from build123d import *

# Parameters (mm, degrees)
F0_R     = 25.4
F1_DEPTH = 12.7
F2_W     = 4.56177
F2_H     = 5.815812
F3_DEPTH = 12.701
F4_R     = 4.759949
F5_DEPTH = 12.701


with BuildPart() as f1:
    # F0 (on Top) → F1 (new body)
    with BuildSketch(Plane.XY):
        Circle(F0_R)
    extrude(amount=F1_DEPTH)

    # F2 (on face) → F3 (cut, through all)
    with BuildSketch(Plane.XY.offset(12.7)):
        with Locations((-10.897615, -5.573769)):
            Rectangle(F2_W, F2_H)
    extrude(amount=-F3_DEPTH, mode=Mode.SUBTRACT)

    # F4 (on face) → F5 (cut, through all)
    with BuildSketch(Plane(origin=(0, 0, 0), x_dir=(1, 0, 0), z_dir=(0, 0, -1))):
        with Locations((8.635784, 2.300633)):
            Circle(F4_R)
    extrude(amount=-F5_DEPTH, mode=Mode.SUBTRACT)


solid = f1.part
Verification items for the finished model (mm, model axes). A direction names the side the tool comes from. Coordinates: 2 decimals unless noted, no trailing zeros. Order: outer loops, then holes, each group sorted by start corner. A loop starts at its lowest first (then second) coordinate and runs counter-clockwise, first axis right, second up. Notation, with made-up numbers: M -17.75,44.5 L 7.25,44.5 A10 ccw 7.25,49.5 Z; hole C 60.5,-10.75 d5. An arc over 180 degrees is marked long. Write each question's results on one line, items separated by ' | '.
1) Section check D-D on x = -20. Record the cut outline in (y, z).
Solved:
outline: M -15.66,0 L 15.66,0 L 15.66,12.7 L -15.66,12.7 Z
2) Section check C-C on y = -21.5. Record the cut outline in (x, z).
Solved:
outline: M -13.52,0 L 13.52,0 L 13.52,12.7 L -13.52,12.7 Z
3) Section check A-A on y = 0. Record the cut outline in (x, z), plus the area to 3 significant figures.
Solved:
outline: M -25.4,0 L 4.47,0 L 4.47,12.7 L -25.4,12.7 Z; M 12.8,0 L 25.4,0 L 25.4,12.7 L 12.8,12.7 Z | area: 539 mm²
4) Access from +Z, -Z, +X, -X, +Y, -Y to the whole of each face (thin tool, end or side, straight path). Record for faces 1 (the face through (0, 0, 0)), 2 (the face through (-13.178, -6, 6)).
Solved:
face 1: -Z, +X, -X, +Y, -Y | face 2: +Z, -Z
5) Scan lines: line 1 along X through (y, z) = (-4.5, 11.75); line 2 along Y through (x, z) = (-10, 1.75); line 3 along Y through (x, z) = (10.5, 8). Record each from-to range of solid material in increasing order. Write a range as [from, to].
Solved:
line 1: x = [-25, -13.18], [-8.62, 4.41], [12.86, 25] | line 2: y = [-23.35, -8.48], [-2.67, 23.35] | line 3: y = [-23.13, -6.68], [2.08, 23.13]
6) Gauge pin test, flat ends, axial feed: pin 1 Ø1.7 at (y, z) = (-4.5, 5) entering from +X; pin 2 Ø6 at (x, z) = (9.5, 2.5) entering from -Y; pin 3 Ø5 at (x, z) = (-11, 4) entering from +Y. Record the tip position at first contact, or that the pin passes through.
Solved:
pin 1: stops at x = 25.14 | pin 2: stops at y = -24.55 | pin 3: stops at y = 23.94
7) Section check B-B on z = 10.75. Record the cut outline in (x, y), plus the area to 3 significant figures.
Solved:
outline: C 0,0 d50.8; hole M -13.18,-8.48 L -8.62,-8.48 L -8.62,-2.67 L -13.18,-2.67 Z; hole C 8.64,-2.3 d9.52 | area: 1,930 mm²
8) Release check for a two-part mould opening along X. For faces 3 (the face through (0, 0, 12.7)), 4 (the face through (-5.506, -24.796, 6.261)), 5 (the face through (-11, -2.666, 6)) record: pulls with the +X half, pulls with the -X half, needs draft (parallel to the pull), parting line crosses it, or undercut.
Solved:
face 3: needs draft | face 4: parting line crosses it | face 5: undercut
